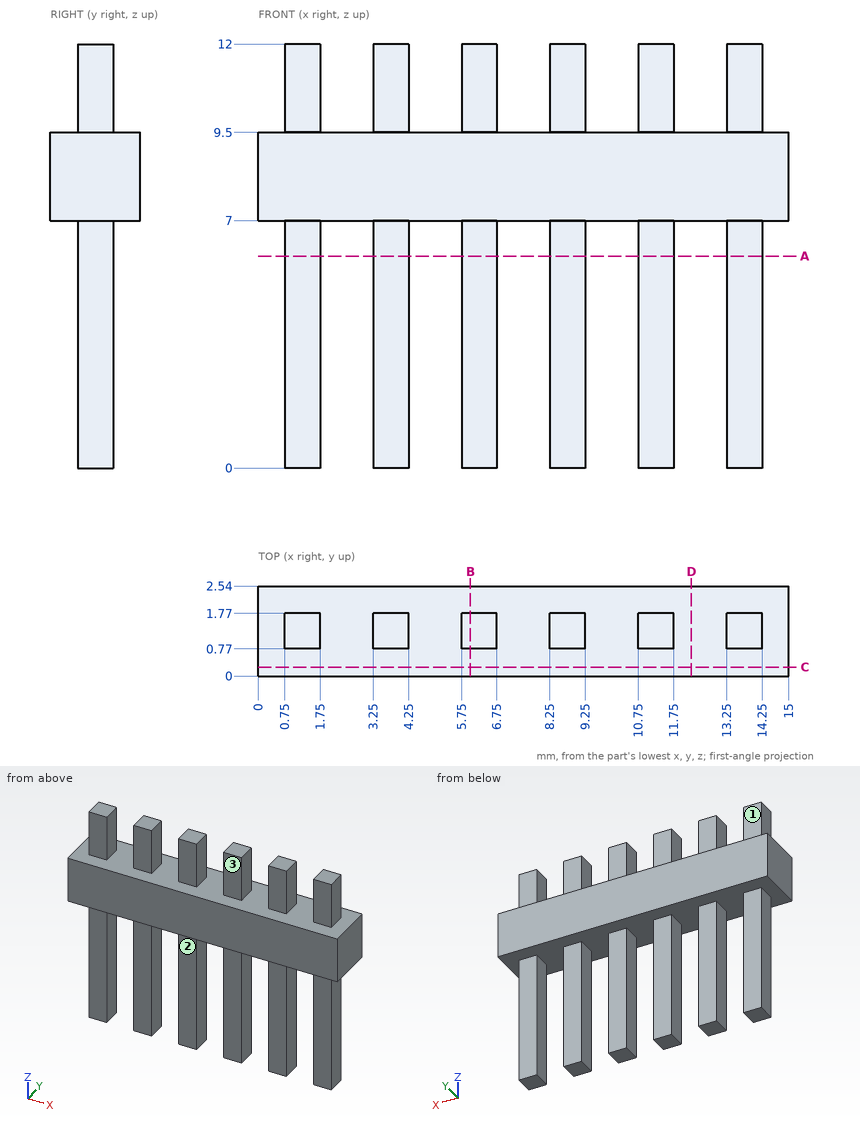
Geometry: see drawing. Coordinates: mm, zero at the bounding-box minimum. A direction names the side the tool comes from. Coordinates: 2 decimals unless noted, no trailing zeros. Loops run counter-clockwise (first coordinate to the right, second up) from the corner with the lowest first, then second, coordinate; pieces in that order, holes last. Notation, with made-up numbers: M 19.5,-27.5 L 24.5,-27.5 A20 ccw 24.5,10.5 Z; hole C 69.25,21.25 d8. An arc over 180 degrees is marked long. Put each result on its own line as item: value. Start each with the question number.
1) Cut plane C-C on y = 0.25. Return the cut outline in (x, z), then the cut area to 3 significant figures.
2) Cut plane B-B on x = 6. Return the cut outline in (y, z).
3) Reachability of the marked faces 1, 2 and 3 from +Z, -Z, +X, -X, +Y, -Y: full face, straight path, thin tool, end or side. Return the list, or none.
4) Cut plane A-A on z = 6. Return the cut outline in (x, y), then the cut area to 3 significant figures.
5) Cut plane D-D on x = 12.25. Return the cut outline in (y, z), then the cut area to 3 significant figures.
6) Ray query, L1, parallel to X at y = 1.45, z = 5.25; L2, parallel to Z at x = 5.5, y = 2.45; L3, parallel to Y at x = 3.5, z = 2.25. Return the intervals inside material, ascending. Write a range as from..to.
7) Contact query for flat-ended pins moving along their axis: pin 1 Ø1.1 at (y, z) = (1.5, 10.5) entering from +X; pin 2 Ø1.1 at (y, z) = (1, 2.5) entering from -X; pin 3 Ø1.1 at (x, z) = (11, 3) entering from +Y. Output: stop coordinate, or through.
The answers:
1. outline: M 0,7 L 15,7 L 15,9.5 L 0,9.5 Z
1. area: 37.5 mm²
2. outline: M 0,7 L 0.77,7 L 0.77,0 L 1.77,0 L 1.77,7 L 2.54,7 L 2.54,9.5 L 1.77,9.5 L 1.77,12 L 0.77,12 L 0.77,9.5 L 0,9.5 Z
3. face 1: +Z, +X, -X, +Y
3. face 2: -Z, +X, -X, -Y
3. face 3: +Z, +X, -X, -Y
4. outline: M 0.75,0.77 L 1.75,0.77 L 1.75,1.77 L 0.75,1.77 Z; M 3.25,0.77 L 4.25,0.77 L 4.25,1.77 L 3.25,1.77 Z; M 5.75,0.77 L 6.75,0.77 L 6.75,1.77 L 5.75,1.77 Z; M 8.25,0.77 L 9.25,0.77 L 9.25,1.77 L 8.25,1.77 Z; M 10.75,0.77 L 11.75,0.77 L 11.75,1.77 L 10.75,1.77 Z; M 13.25,0.77 L 14.25,0.77 L 14.25,1.77 L 13.25,1.77 Z
4. area: 6.00 mm²
5. outline: M 0,7 L 2.54,7 L 2.54,9.5 L 0,9.5 Z
5. area: 6.35 mm²
6. L1: x = 0.75..1.75, 3.25..4.25, 5.75..6.75, 8.25..9.25, 10.75..11.75, 13.25..14.25
6. L2: z = 7..9.5
6. L3: y = 0.77..1.77
7. pin 1: stops at x = 14.25
7. pin 2: stops at x = 0.75
7. pin 3: stops at y = 1.77
